Geometry: see drawing. Coordinates: mm, zero at the bounding-box minimum. A direction names the side the tool comes from. Coordinates: 2 decimals unless noted, no trailing zeros. Write each loop counter-clockwise with the first axis right and the second up, starting at its lowest first coordinate (ties: lowest second). Pieces come first, ordered by that corner, then holes.
1) Line query: L1, parallel to Y at x = 15, z = 4; L2, parallel to Y at x = 15, z = 10.4; L3, parallel to Z at x = 17.5, y = 28. Output: solid intervals per line, ascending.
2) Section query C-C (y = 5). Output: boundary loops of the cut face in (x, z).
3) Section query B-B (y = 15). Output: boundary loops of the cut face in (x, z), then the cut area to 3 significant figures.
4) Set-up query: the marked faces 5 and 6. Return all of +Z, -Z, +X, -X, +Y, -Y with unobstructed straight access to the full face (end or side cutting, diameter ignored); none if empty.
5) Section query A-A (x = 15). Output: boundary loops of the cut face in (y, z).
6) Section query D-D (z = 5.5). Output: boundary loops of the cut face in (x, y), then the cut area to 3 significant figures.
7) Pin query (flat end, axial travel): pin 1 Ø3 at (x, z) = (21, 10.5) entering from +Y (1 decimal); pin 2 Ø12 at (x, y) = (5.5, 36.5) entering from +Z; pin 3 Ø5 at (y, z) = (52, 3) entering from +X. Return the tip coordinate at first contact, or that it passes through.
8) Draft query along X for the marked faces 1, 2, 3 and 4. Return one class per face: pulls with the +X half, pulls with the -X half, needs draft (parallel to the pull), parting line crosses it, or undercut.
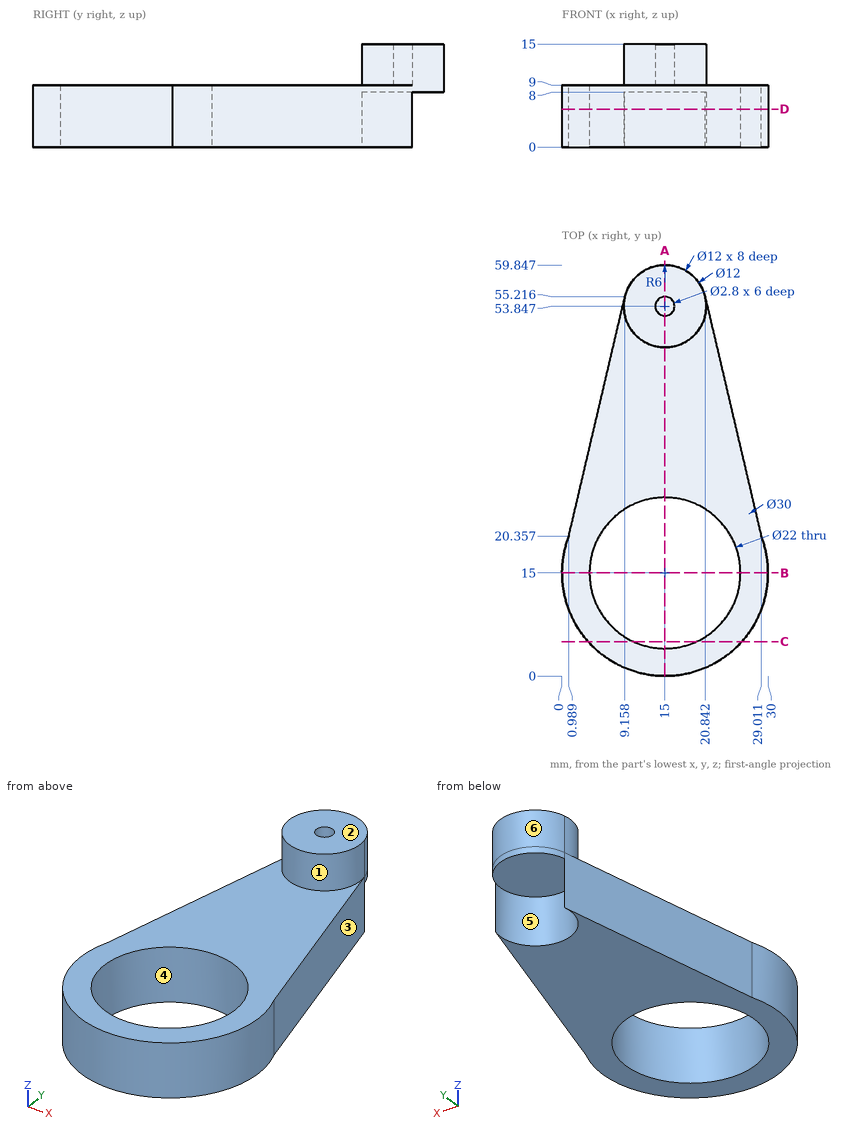
Answer:
1. L1: y = 0 to 4, 26 to 47.85
1. L2: y = 47.85 to 52.45, 55.25 to 59.85
1. L3: z = 0 to 9
2. outline: (3.82, 0) - (10.42, 0) - (10.42, 9) - (3.82, 9) - close; (19.58, 0) - (26.18, 0) - (26.18, 9) - (19.58, 9) - close
3. outline: (0, 0) - (4, 0) - (4, 9) - (0, 9) - close; (26, 0) - (30, 0) - (30, 9) - (26, 9) - close
3. area: 72.0 mm2
4. face 5: -Z
4. face 6: +Z, -Z, +Y
5. outline: (0, 0) - (4, 0) - (4, 9) - (0, 9) - close; (26, 0) - (47.85, 0) - (47.85, 8) - (59.85, 8) - (59.85, 15) - (55.25, 15) - (55.25, 9) - (52.45, 9) - (52.45, 15) - (47.85, 15) - (47.85, 9) - (26, 9) - close
6. outline: (0.99, 20.36) arc R15 ccw (long way) to (29.01, 20.36) - (20.85, 55.2) arc R6 cw (long way) to (9.15, 55.2) - close; hole circle Ø22 at (15, 15)
6. area: 750 mm2
7. pin 1: stops at y = 57.8
7. pin 2: stops at z = 9
7. pin 3: stops at x = 22.18
8. face 1: parting line crosses it
8. face 2: needs draft
8. face 3: pulls with the +X half
8. face 4: undercut
